```python
from build123d import *

# Parameters (mm, degrees)
F0_W     = 139
F0_H     = 209
F0_W_2   = 125
F0_H_2   = 195
F1_DEPTH = 20
F2_DEPTH = 5
F3_W     = 45
F3_H     = 35
F4_DEPTH = 15
F5_R     = 6.5
F6_DEPTH = 25
F7_R     = 5
F9_DEPTH = 5


with BuildPart() as f1:
    # F0 (on Top) → F1 (new body)
    with BuildSketch(Plane.XY):
        with Locations((62.5, 97.5)):
            Rectangle(F0_W, F0_H)
        with Locations((62.5, 97.5)):
            Rectangle(F0_W_2, F0_H_2, mode=Mode.SUBTRACT)
        with Locations((62.5, 97.5)):
            Rectangle(F0_W_2, F0_H_2)
    extrude(amount=-F1_DEPTH)

    # F0 (on Top) → F2 (cut)
    with BuildSketch(Plane.XY):
        with Locations((62.5, 97.5)):
            Rectangle(F0_W_2, F0_H_2)
    extrude(amount=-F2_DEPTH, mode=Mode.SUBTRACT)

    # F3 (on face) → F4 (cut)
    with BuildSketch(Plane.XY):
        with Locations((62.5, 32.5)):
            Rectangle(F3_W, F3_H)
    extrude(amount=-F4_DEPTH, mode=Mode.SUBTRACT)

    # F5 (on face) → F6 (cut)
    with BuildSketch(Plane.XY):
        with Locations((62.5, 32.5)):
            Circle(F5_R)
    extrude(amount=-F6_DEPTH, mode=Mode.SUBTRACT)

    # F7
    f7_edges = [f1.edges().sort_by_distance(p)[0] for p in [
        (-7, -7, -10),
        (125, 195, -2.5),
        (-7, 202, -10),
        (132, -7, -10),
        (132, 202, -10),
    ]]
    fillet(f7_edges, radius=F7_R)

    # F8 (on face) → F9 (join)
    with BuildSketch(Plane(origin=(0, 0, -20), x_dir=(1, 0, 0), z_dir=(0, 0, -1))):
        Polygon((-27, -170), (-7, -170), (-7, -160), (-17, -160), (-17, -120), (-7, -120), (-7, -110), (-27, -110), align=None)
        Polygon((-27, -78), (-7, -78), (-7, -68), (-17, -68), (-17, -28), (-7, -28), (-7, -18), (-27, -18), align=None)
        Polygon((132, -68), (132, -78), (152, -78), (152, -18), (132, -18), (132, -28), (142, -28), (142, -68), align=None)
        Polygon((132, -170), (152, -170), (152, -110), (132, -110), (132, -120), (142, -120), (142, -160), (132, -160), align=None)
    extrude(amount=-F9_DEPTH)


solid = f1.part
```
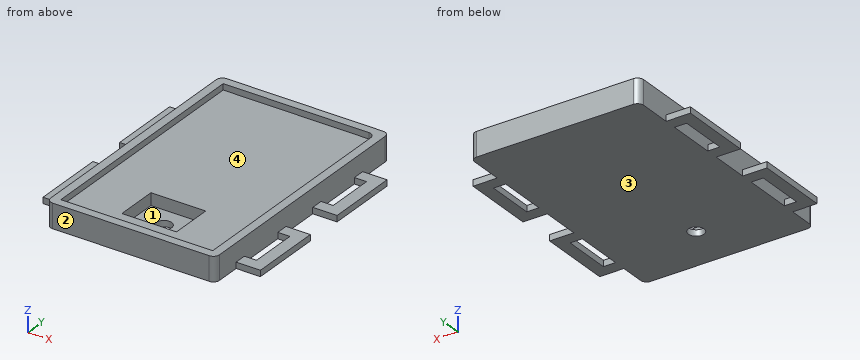
Model file for the job. Use its own axes, mm. Face numbers are marked on the shaded views. A direction names the side the tool comes from. Coordinates: 2 decimals unless noted, no trailing zeros. Loops run counter-clockwise (first coordinate to the right, second up) from the corner with the lowest first, then second, coordinate; pieces in that order, holes last. Notation, with made-up numbers: (35, 66.5) -> (87, 66.5) arc R36 ccw to (87, 101.5) -> close; hole circle Ø1 at (-36.5, 5.25). An arc over 180 degrees is marked (long way). Answer as a JSON object with one key per item and string values.
Q1. Pull direction X, two halves, no side cores. Call the marked faces 1 and 2: released by +X, released by -X, zero draft, split by the parting line, or undercut.
Report:
{"face 1": "undercut", "face 2": "zero draft"}
Q2. Cut at C-C (z = -2.5). List the corners of the cut face in (x, y).
Report:
{"outline": "(-7, -2) arc R5 ccw to (-2, -7) -> (127, -7) arc R5 ccw to (132, -2) -> (132, 197) arc R5 ccw to (127, 202) -> (-2, 202) arc R5 ccw to (-7, 197) -> close; hole (0, 0) -> (125, 0) -> (125, 190) arc R5 ccw to (120, 195) -> (0, 195) -> close"}
Q3. Cut at B-B (y = 53.5). List the corners of the cut face in (x, z).
Report:
{"outline": "(-27, -20) -> (-17, -20) -> (-17, -15) -> (-27, -15) -> close; (-7, -20) -> (132, -20) -> (132, 0) -> (125, 0) -> (125, -5) -> (0, -5) -> (0, 0) -> (-7, 0) -> close; (142, -20) -> (152, -20) -> (152, -15) -> (142, -15) -> close"}
Q4. Flat gauge pins, fed straight in: P1, Ø4, axis at y = 133, z = -2.5, coming from the -X side; P2, Ø2, axis at x = -9, z = -9, coming from the +Y side; P3, Ø5.5, axis at x = 139.5, z = -18, coming from the +Y side; P4, Ø10.5, axis at x = 63.5, y = 40, coming from the +Z side. Where does each tip first touch, or does it go through?
Report:
{"P1": "stops at x = -7", "P2": "passes through", "P3": "stops at y = 170", "P4": "stops at z = -15"}
Q5. 3-axis set-ups, long thin cutter, end or side, ignore diameter. For the marked faces 3 and 4: which of +Z, -Z, +X, -X, +Y, -Y reach the whole face in a straight line?
Report:
{"face 3": "-Z, +X, -X, +Y, -Y", "face 4": "+Z"}
Q6. Probe probe 1 along X at (y, z) = (33.5, -9.5); probe 2 along Y at (x, z) = (62.5, -16); probe 3 along X at (y, z) = (130, -3.75). List the from-to ranges inside material, lowest first.
Report:
{"probe 1": "x = -7 to 40, 85 to 132", "probe 2": "y = -7 to 26, 39 to 202", "probe 3": "x = -7 to 0, 125 to 132"}
Q7. Cut at D-D (x = 62.5). List the corners of the cut face in (y, z).
Report:
{"outline": "(-7, -20) -> (26, -20) -> (26, -15) -> (15, -15) -> (15, -5) -> (0, -5) -> (0, 0) -> (-7, 0) -> close; (39, -20) -> (202, -20) -> (202, 0) -> (195, 0) -> (195, -5) -> (50, -5) -> (50, -15) -> (39, -15) -> close"}
Q8. Cut at A-A (y = 32.5). List the corners of the cut face in (x, z).
Report:
{"outline": "(-27, -20) -> (-17, -20) -> (-17, -15) -> (-27, -15) -> close; (-7, -20) -> (56, -20) -> (56, -15) -> (40, -15) -> (40, -5) -> (0, -5) -> (0, 0) -> (-7, 0) -> close; (69, -20) -> (132, -20) -> (132, 0) -> (125, 0) -> (125, -5) -> (85, -5) -> (85, -15) -> (69, -15) -> close; (142, -20) -> (152, -20) -> (152, -15) -> (142, -15) -> close"}
